```python
from build123d import *

# Parameters (mm, degrees)
SKETCH1_W           = 50.8
SKETCH1_H           = 38.1
BOSS_EXTRUDE1_DEPTH = 5.08
SKETCH2_W           = 16.51
SKETCH2_H           = 10.16
BOSS_EXTRUDE2_DEPTH = 76.2
SKETCH3_W           = 3.81
SKETCH3_H           = 10.16
CUT_EXTRUDE1_DEPTH  = 76.2
SKETCH4_W           = 16.51
SKETCH4_H           = 10.16
BOSS_EXTRUDE3_DEPTH = 12.7
SKETCH6_W           = 16.51
SKETCH6_H           = 12.7
CUT_EXTRUDE2_DEPTH  = 3.81
SKETCH5_R           = 3.683
BOSS_EXTRUDE4_DEPTH = 3.81
FILLET1_R           = 7.62
FILLET4_R           = 7.62
FILLET7_R           = 7.62


with BuildPart() as part:
    # Sketch1 → Boss-Extrude1 (new body)
    with BuildSketch(Plane.XY):
        Rectangle(SKETCH1_W, SKETCH1_H)
    extrude(amount=BOSS_EXTRUDE1_DEPTH)

    # Sketch2 → Boss-Extrude2 (add)
    with BuildSketch(Plane.XY.offset(5.08)):
        with Locations((-13.335, -5.842)):
            Rectangle(SKETCH2_W, SKETCH2_H)
        with Locations((13.335, -5.842)):
            Rectangle(SKETCH2_W, SKETCH2_H)
    extrude(amount=BOSS_EXTRUDE2_DEPTH)

    # Sketch3 → Cut-Extrude1 (cut)
    with BuildSketch(Plane.XY.offset(81.28)):
        with Locations((-6.985, -5.842)):
            Rectangle(SKETCH3_W, SKETCH3_H)
        with Locations((6.985, -5.842)):
            Rectangle(SKETCH3_W, SKETCH3_H)
    extrude(amount=-CUT_EXTRUDE1_DEPTH, mode=Mode.SUBTRACT)

    # Sketch4 → Boss-Extrude3 (add)
    with BuildSketch(Plane.XY.offset(81.28)):
        with Locations((-13.335, -5.842)):
            Rectangle(SKETCH4_W, SKETCH4_H)
        with Locations((13.335, -5.842)):
            Rectangle(SKETCH4_W, SKETCH4_H)
    extrude(amount=BOSS_EXTRUDE3_DEPTH)

    # Sketch6 → Cut-Extrude2 (cut)
    with BuildSketch(Plane.XZ.offset(10.922)):
        with Locations((-13.335, 87.63)):
            Rectangle(SKETCH6_W, SKETCH6_H)
        with Locations((13.335, 87.63)):
            Rectangle(SKETCH6_W, SKETCH6_H)
    extrude(amount=-CUT_EXTRUDE2_DEPTH, mode=Mode.SUBTRACT)

    # Sketch5 → Boss-Extrude4 (add)
    with BuildSketch(Plane.XZ.offset(10.922)):
        with Locations(Location((-13.335, 87.63, 0), (0, 0, 270))):
            Circle(SKETCH5_R)
        with Locations(Location((13.335, 87.63, 0), (0, 0, 270))):
            Circle(SKETCH5_R)
    extrude(amount=-BOSS_EXTRUDE4_DEPTH)

    # Fillet1
    # the kernel refuses this fillet: 7.62 mm, written as the material it takes off along each edge
    with BuildSketch(Plane(origin=(-43.360512242, 19.05, 0), x_dir=(0, -1, 0), z_dir=(1, 0, 0))) as fillet1_piece_1:
        with BuildLine():
            CenterArc((7.184204897, -7.62), FILLET1_R, 90, 70.528779366)
            Line((0, -5.08), (-0.143684098, -5.0292))
            ThreePointArc((-0.143684098, -5.0292), (-0.1524, -2.54), (-0.1524, 0))
            Line((-0.1524, 0), (0, 0.1524))
            Line((0, 0.1524), (7.184204897, 0.1524))
            Line((7.184204897, 0.1524), (7.184204897, 0))
        make_face()
    extrude(amount=86.721024484, mode=Mode.SUBTRACT)

    # Fillet4
    # the kernel refuses this fillet: 7.62 mm, written as the material it takes off along each edge
    with BuildSketch(Plane(origin=(-25.4, -37.010512242, 0), x_dir=(0, 0, 1), z_dir=(0, 1, 0)), Plane(origin=(25.4, 29.826307345, 0), x_dir=(0, 0, 1), z_dir=(0, -1, 0))) as fillet4_piece_1:
        with BuildLine():
            CenterArc((7.62, 7.184204897), FILLET4_R, 180, 70.528779366)
            Line((0, 7.184204897), (-0.1524, 7.184204897))
            Line((-0.1524, 7.184204897), (-0.1524, 0))
            Line((-0.1524, 0), (0, -0.1524))
            ThreePointArc((0, -0.1524), (2.54, -0.1524), (5.0292, -0.143684098))
            Line((5.0292, -0.143684098), (5.08, 0))
        make_face()
    extrude(amount=66.836819587, mode=Mode.SUBTRACT)

    # Fillet7
    # the kernel refuses this fillet: 7.62 mm, written as the material it takes off along each edge
    with BuildSketch(Plane(origin=(-18.215795103, -19.05, 7.62), x_dir=(0.5563472554155052, 0, 0.8309498970405103), z_dir=(0.8309498970405103, 0, -0.5563472554155052))) as fillet7_piece_1:
        with BuildLine():
            CenterArc((7.62 - FILLET7_R, -FILLET7_R), FILLET7_R, 0, 90)
            Line((7.62, -FILLET7_R), (7.62, 0))
            Line((7.62, 0), (7.62 - FILLET7_R, 0))
        make_face()
    revolve(axis=Axis((-18.215795103, -19.05, 7.62), (0, -1, 0)), revolution_arc=213.803560609, mode=Mode.SUBTRACT)
    with BuildSketch(Plane(origin=(18.215795103, -19.05, 7.62), x_dir=(-0.5563472554155037, 0, 0.8309498970405114), z_dir=(-0.8309498970405114, 0, -0.5563472554155037))) as fillet7_piece_2:
        with BuildLine():
            CenterArc((7.62 - FILLET7_R, FILLET7_R), FILLET7_R, 270, 90)
            Line((7.62, FILLET7_R), (7.62, 0))
            Line((7.62, 0), (7.62 - FILLET7_R, 0))
        make_face()
    revolve(axis=Axis((18.215795103, -19.05, 7.62), (0, 1, 0)), revolution_arc=213.803560609, mode=Mode.SUBTRACT)
    with BuildSketch(Plane(origin=(18.215795103, -19.05, 0), x_dir=(0, 0, 1), z_dir=(-1, 0, 0))) as fillet7_piece_3:
        with BuildLine():
            CenterArc((FILLET7_R, FILLET7_R), FILLET7_R, 180, 90)
            Line((0, FILLET7_R), (0, 0))
            Line((0, 0), (FILLET7_R, 0))
        make_face()
    extrude(amount=36.431590206, mode=Mode.SUBTRACT)


solid = part.part
```
The model under review builds one solid part; all positions refer to its coordinate system, in mm. A direction names the side the tool comes from. Round coordinates to 2 decimals unless told otherwise and drop trailing zeros. Order: outer loops, then holes, each group sorted by start corner. A loop starts at its lowest first (then second) coordinate and runs counter-clockwise, first axis right, second up. Notation, with made-up numbers: (64.25, -32.75) -> (79.25, -32.75) arc R25 ccw to (79.25, -13.75) -> close; hole circle Ø5 at (4.25, 74.5). An arc over 180 degrees is marked (long way). Use a Markdown table: item, result.
Q1. For line 1 (Z direction, x = 6, y = -5.5); line 2 (Y direction, x = 14.5, z = 76); line 3 (Z direction, x = 2.5, y = 10), list the stretches that pass through material, from the lowest coordinate up.
Values:
| item | result |
|---|---|
| line 1 | z = 0 to 5.08, 81.28 to 93.98 |
| line 2 | y = -10.92 to -0.76 |
| line 3 | z = 0 to 5.08 |
Q2. Clearance check with flat-ended pins moving along their axes: P1, Ø5, axis at y = -6.5, z = 13.5, coming from the -X side; P2, Ø2, axis at x = 12.5, z = 88, coming from the -Y side; P3, Ø5, axis at y = -4.5, z = 55.5, coming from the +X side; P4, Ø3, axis at x = -6, z = 39, coming from the -Y side. State where each tip first meets the part, or that it passes through.
Values:
| item | result |
|---|---|
| P1 | stops at x = -21.59 |
| P2 | stops at y = -10.92 |
| P3 | stops at x = 21.59 |
| P4 | passes through |
Q3. Tool access review of faces 5 (the flat face through (15, -9, 81.28)), 6 (the flat face through (8.89, -6, 44)), 7 (the flat face through (-5.08, -4, 88)), 8 (the flat face through (-13, -10.922, 88)): name each direction out of +Z, -Z, +X, -X, +Y, -Y from which nothing blocks a thin tool from reaching the whole face with its end or side.
Values:
| item | result |
|---|---|
| face 5 | +X, -X, -Y |
| face 6 | +Y, -Y |
| face 7 | +Z, +Y, -Y |
| face 8 | +Z, +X, -X, -Y |
Q4. We need section B-B on y = -3.5. Write out the cut boundary in (x, z), then the cut area to 3 significant figures.
Values:
| item | result |
|---|---|
| outline | (-25.4, 5.08) arc R7.62 ccw to (-18.22, 0) -> (18.22, 0) arc R7.62 ccw to (25.4, 5.08) -> (21.59, 5.08) -> (21.59, 93.98) -> (5.08, 93.98) -> (5.08, 81.28) -> (8.89, 81.28) -> (8.89, 5.08) -> (-8.89, 5.08) -> (-8.89, 81.28) -> (-5.08, 81.28) -> (-5.08, 93.98) -> (-21.59, 93.98) -> (-21.59, 5.08) -> close |
| area | 2,590 mm^2 |
Q5. We need section D-D on x = 16. Write out the cut boundary in (y, z).
Values:
| item | result |
|---|---|
| outline | (-18.61, 5.08) arc R7.62 ccw to (-11.43, 0) -> (11.87, 0) arc R7.62 ccw to (19.05, 5.08) -> (-0.76, 5.08) -> (-0.76, 93.98) -> (-7.11, 93.98) -> (-7.11, 90.17) -> (-10.92, 90.17) -> (-10.92, 85.09) -> (-7.11, 85.09) -> (-7.11, 81.28) -> (-10.92, 81.28) -> (-10.92, 5.08) -> close |
Q6. We need section A-A on z = 87.63. Write out the cut boundary in (x, y).
Values:
| item | result |
|---|---|
| outline | (-21.59, -7.11) -> (-17.02, -7.11) -> (-17.02, -10.92) -> (-9.65, -10.92) -> (-9.65, -7.11) -> (-5.08, -7.11) -> (-5.08, -0.76) -> (-21.59, -0.76) -> close; (5.08, -7.11) -> (9.65, -7.11) -> (9.65, -10.92) -> (17.02, -10.92) -> (17.02, -7.11) -> (21.59, -7.11) -> (21.59, -0.76) -> (5.08, -0.76) -> close |
Q7. We need section C-C on z = 78. Write out the cut boundary in (x, y).
Values:
| item | result |
|---|---|
| outline | (-21.59, -10.92) -> (-8.89, -10.92) -> (-8.89, -0.76) -> (-21.59, -0.76) -> close; (8.89, -10.92) -> (21.59, -10.92) -> (21.59, -0.76) -> (8.89, -0.76) -> close |
Q8. Mouldability with a two-part tool opening along Z and no side actions: class faces 1 (the flat face through (-7, -4, 81.28)), 2 (the flat face through (15, -0.762, 49)), 3 (the flat face through (-8.89, -6, 44)), 4 (the cylindrical face through (-22.56, 3.6, 1.36)) as +Z half, -Z half, draft (parallel to the pull), parting line (faces both ways), or undercut.
Values:
| item | result |
|---|---|
| face 1 | undercut |
| face 2 | draft |
| face 3 | undercut |
| face 4 | -Z half |
